Source: CAD feature listing. Evaluate the final solid. Frame: model axes, mm. Round coordinates to 2 decimals unless told otherwise and drop trailing zeros. Order: outer loops, then holes, each group sorted by start corner. A loop starts at its lowest first (then second) coordinate and runs counter-clockwise, first axis right, second up. Notation, with made-up numbers: (64.25, 26) - (82.25, 26) arc R21 cw to (82.25, 65) - close; hole circle Ø5 at (-9.75, 11.5). An arc over 180 degrees is marked (long way). Use one line per item in the form item = value. Start each with the question number.
Q1. Cut plane B-B, the plane z = 1.5. Return the cut outline in (x, y).
Q2. Cut plane C-C, the plane x = 110.75. Return the cut outline in (y, z).
Q3. Cut plane A-A, the plane y = 12.75. Return the cut outline in (x, z), and give its area (4 significant figures).
Q4. Ray query, line 1 (Y direction, x = 152.75, z = 1); line 2 (X direction, y = 32, z = 1.3); line 3 (Y direction, x = 82.75, z = 2.4). Return the intervals inside material, ascending. Write a range as [from, to].
Q5. Pin query (flat end, axial travel): pin 1 Ø0.9 at (x, z) = (3, 1.5) entering from +Y; pin 2 Ø1.5 at (y, z) = (41.5, 1.5) entering from +X; pin 3 Ø0.9 at (x, z) = (217.5, 1.5) entering from -Y. Return the tip coordinate at first contact, or that it passes through.
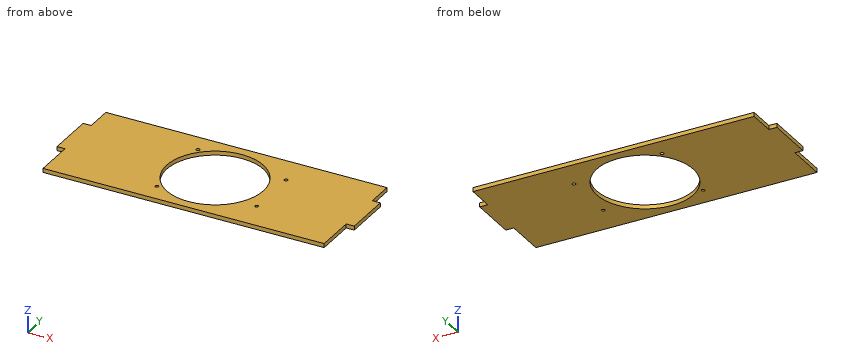
from build123d import *

# Parameters (mm, degrees)
BOSS_EXTRUDE1_DEPTH = 3
SKETCH2_R           = 36
CUT_EXTRUDE1_DEPTH  = 229.367029144
CAVITY1_OUTLINE_R   = 1.25
CAVITY1_DEPTH       = 3


# Read off the part's stored shape, not the designer's step: Cavity1
with BuildPart() as part:
    # Sketch1 → Boss-Extrude1 (new body)
    with BuildSketch(Plane.XY):
        Polygon((6, -30), (215.5, -30), (215.5, 0), (221.5, 0), (221.5, 35.5), (215.5, 35.5), (215.5, 55.5), (6, 55.5), (6, 35.5), (0, 35.5), (0, 0), (6, 0), align=None)
    extrude(amount=BOSS_EXTRUDE1_DEPTH)

    # Sketch2 → Cut-Extrude1 (cut, through all)
    with BuildSketch(Plane.XY.offset(3)):
        with Locations((110.75, 12.75)):
            Circle(SKETCH2_R)
    extrude(amount=-CUT_EXTRUDE1_DEPTH, mode=Mode.SUBTRACT)

    # Cavity1 outline → Cavity1 (cut)
    with BuildSketch(Plane.XY):
        with Locations((152.75, 32.75)):
            Circle(CAVITY1_OUTLINE_R)
        with Locations((152.75, -7.25)):
            Circle(CAVITY1_OUTLINE_R)
        with Locations((82.75, -15.25)):
            Circle(CAVITY1_OUTLINE_R)
        with Locations((82.75, 40.75)):
            Circle(CAVITY1_OUTLINE_R)
    extrude(amount=CAVITY1_DEPTH, mode=Mode.SUBTRACT)


solid = part.part
Completed:
q1.outline = (0, 0) - (6, 0) - (6, -30) - (215.5, -30) - (215.5, 0) - (221.5, 0) - (221.5, 35.5) - (215.5, 35.5) - (215.5, 55.5) - (6, 55.5) - (6, 35.5) - (0, 35.5) - close; hole circle Ø72 at (110.75, 12.75); hole circle Ø2.5 at (82.75, -15.25); hole circle Ø2.5 at (82.75, 40.75); hole circle Ø2.5 at (152.75, -7.25); hole circle Ø2.5 at (152.75, 32.75)
q2.outline = (-30, 0) - (-23.25, 0) - (-23.25, 3) - (-30, 3) - close; (48.75, 0) - (55.5, 0) - (55.5, 3) - (48.75, 3) - close
q3.outline = (0, 0) - (74.75, 0) - (74.75, 3) - (0, 3) - close; (146.75, 0) - (221.5, 0) - (221.5, 3) - (146.75, 3) - close
q3.area = 448.5 mm2
q4.line_1 = [-30, -8.5], [-6, 31.5], [34, 55.5]
q4.line_2 = [0, 80.33], [141.17, 151.75], [153.75, 221.5]
q4.line_3 = [-30, -16.5], [-14, -9.88], [35.38, 39.5], [42, 55.5]
q5.pin_1 = 35.5
q5.pin_2 = 215.5
q5.pin_3 = 0
